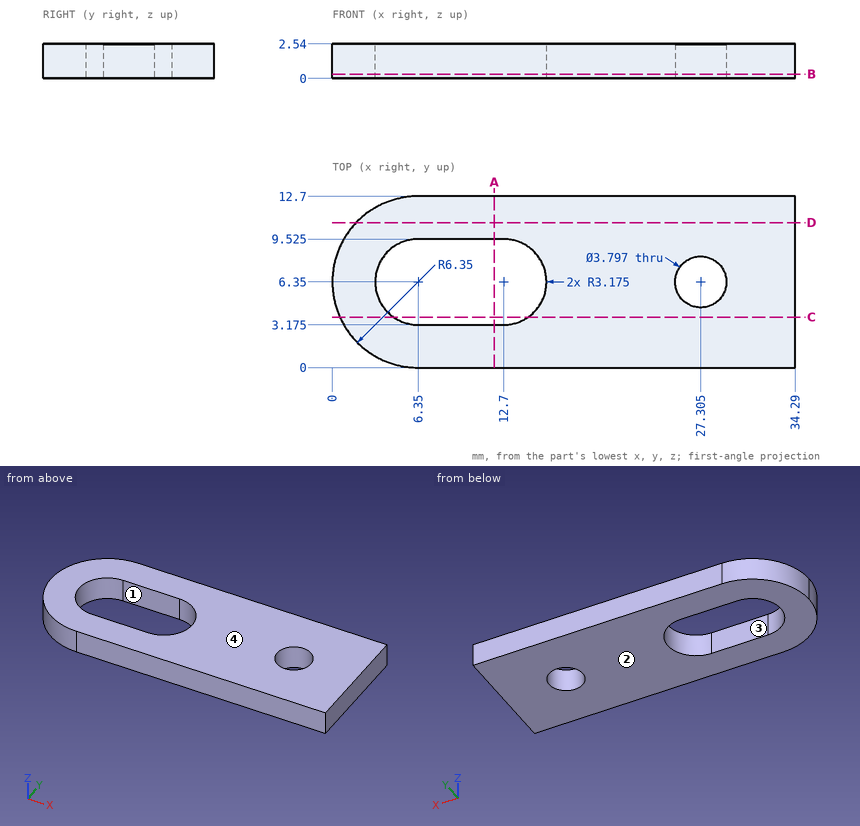
Source: three-view drawing plus pictorial views. Frame: mm from the lowest corner of the part. A direction names the side the tool comes from. Coordinates: 2 decimals unless noted, no trailing zeros. Write each loop counter-clockwise with the first axis right and the second up, starting at its lowest first coordinate (ties: lowest second). Pieces come first, ordered by that corner, then holes. Notation, with made-up numbers: (16, -29.5) -> (54, -29.5) arc R25 cw to (54, 2.5) -> close; hole circle Ø11 at (86.25, 7). An arc over 180 degrees is marked (long way). Answer as a JSON object with one key per item and string values.
1. Section B-B on z = 0.3. Count the separate pieces of the cut face and the enclosed holes in it, then the cut area to 3 significant figures.
Result set:
{"separate pieces": "1", "enclosed holes": "2", "area": "335 mm2"}
2. Section C-C on y = 3.75. Return the cut outline in (x, z), then the cut area to 3 significant figures.
Result set:
{"outline": "(0.56, 0) -> (4.53, 0) -> (4.53, 2.54) -> (0.56, 2.54) -> close; (14.52, 0) -> (34.29, 0) -> (34.29, 2.54) -> (14.52, 2.54) -> close", "area": "60.3 mm2"}
3. Section D-D on y = 10.75. Return the cut outline in (x, z).
Result set:
{"outline": "(1.77, 0) -> (34.29, 0) -> (34.29, 2.54) -> (1.77, 2.54) -> close"}
4. Access query for the marked faces 3 and 4. Directions: +Z, -Z, +X, -X, +Y, -Y. A direction counts if a zero-diameter tool reaches every point of the face in a straight line with its end or side. Return the directions, or none.
Result set:
{"face 3": "+Z, -Z", "face 4": "+Z, +X, -X, +Y, -Y"}
5. Section A-A on x = 12. Return the cut outline in (y, z) (1 decimal), then the cut area to 3 significant figures.
Result set:
{"outline": "(0, 0) -> (3.2, 0) -> (3.2, 2.5) -> (0, 2.5) -> close; (9.5, 0) -> (12.7, 0) -> (12.7, 2.5) -> (9.5, 2.5) -> close", "area": "16.1 mm2"}
6. First-contact query: P1, Ø1, axis at y = 4, z = 1, coming from the -X side (1 decimal). Flat tip, straight axial feed; report the tip coordinate or a pass-through.
Result set:
{"P1": "stops at x = 0.3"}
7. Material intervals for line 1 (X direction, y = 7.5, z = 2.45) (1 decimal); line 2 (Y direction, x = 8, z = 0.4) (1 decimal); line 3 (X direction, y = 6.75, z = 1.3), sorted ascending. Write a range as from..to.
Result set:
{"line 1": "x = 0.1..3.4, 15.7..25.8, 28.8..34.3", "line 2": "y = 0..3.2, 9.5..12.7", "line 3": "x = 0.01..3.2, 15.85..25.45, 29.16..34.29"}
8. Mould query, pull axis X, two halves, no side actions, for the marked faces 1 and 2. Classes: released by +X, released by -X, zero draft, split by the parting line, or undercut.
Result set:
{"face 1": "undercut", "face 2": "zero draft"}
